Autodesk Inventor part; units mm, degrees
ref_plane "YZ Plane" through (0, 0, 0) normal (1, 0, 0) x (0, 1, 0)
ref_plane "XZ Plane" through (0, 0, 0) normal (0, 1, 0) x (-1, 0, 0)
ref_plane "XY Plane" through (0, 0, 0) normal (0, 0, 1) x (1, 0, 0)
sketch "Sketch1" plane through (0, 0, 0) normal (0, 0, 1) x (1, 0, 0)
  circle A0 centre (0, 0) radius 2.65
  circle A1 centre (0, 0) radius 3.5
  dimension "d0" = 5.3
  dimension "d1" = 7
extrude "Extrusion1" add sketch "Sketch1" along normal blind 15
sketch "Sketch2" plane through (0, 0, 15) normal (0, 0, 1) x (1, 0, 0)
  circle A0 centre (0, 0) radius 2.65
  circle A1 centre (0, 0) radius 3.75
  line L0 (-6, 0.85) -> (6, 0.85)
  line L1 (6, 0.85) -> (6, -0.85)
  line L2 (6, -0.85) -> (-6, -0.85)
  line L3 (-6, -0.85) -> (-6, 0.85)
  line L4 (-6, 0.85) -> (6, -0.85) construction
  line L5 (6, 0.85) -> (-6, -0.85) construction
  point P0 (-3.6524, 0.85)
  point P1 (-3.6524, -0.85)
  point P2 (3.6524, -0.85)
  point P3 (3.6524, 0.85)
  dimension "d4" = 7.5
  dimension "d5" = 12
  dimension "d6" = 1.7
extrude "Extrusion2" add sketch "Sketch2" along normal blind 25 contours A0 L0 A1 L2 | A0 L0 A1 | L2 A1 A0 | A0 L2 A1 L0 | L0 L1 L2 A1 | A1 L2 L3 L0
properties part number "final pin_3DPrint"
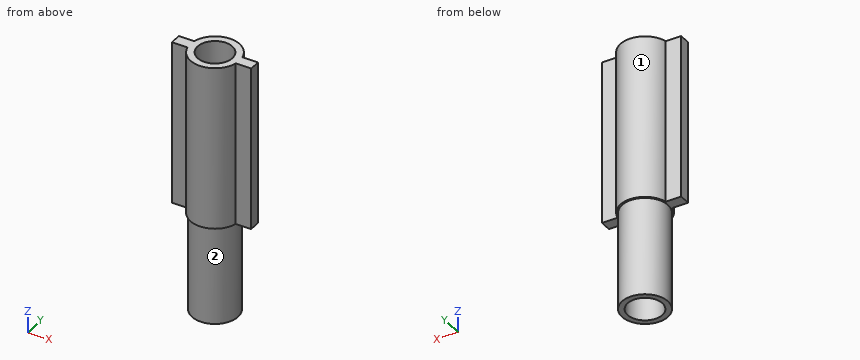
Could you check a few things on this model? Use its own coordinates, in mm. Face numbers are marked on the shaded views. A direction names the side the tool comes from. Round coordinates to 2 decimals unless told otherwise and drop trailing zeros. Order: outer loops, then holes, each group sorted by start corner. A loop starts at its lowest first (then second) coordinate and runs counter-clockwise, first axis right, second up.
(1) Imagine slicing it at A-A (y = 0). Write out the boundary of the cut face in (x, z).
Response values:
outline: (-6, 15) - (-3.5, 15) - (-3.5, 0) - (-2.65, 0) - (-2.65, 40) - (-6, 40) - close; (2.65, 0) - (3.5, 0) - (3.5, 15) - (6, 15) - (6, 40) - (2.65, 40) - close
(2) I'm going to push flat-ended pins straight in: pin 1 (3 mm diameter, centred on x = -1.5, z = 25.5, fed in from +Y); pin 2 (2 mm diameter, centred on x = 0.5, y = 1, fed in from -Z); pin 3 (0.7 mm diameter, centred on x = -4.5, z = 21.5, fed in from -Y); pin 4 (1.2 mm diameter, centred on x = -4.5, z = 25.5, fed in from +Y). Where does each tip first touch, or does it pass through?
Response values:
pin 1: stops at y = 3.75
pin 2: passes through
pin 3: stops at y = -0.85
pin 4: stops at y = 0.85
(3) Imagine slicing it at C-C (z = 21). Write out the boundary of the cut face in (x, y).
Response values:
outline: (-6, -0.85) - (-3.65, -0.85) arc R3.75 ccw to (3.65, -0.85) - (6, -0.85) - (6, 0.85) - (3.65, 0.85) arc R3.75 ccw to (-3.65, 0.85) - (-6, 0.85) - close; hole circle Ø5.3 at (0, 0)
(4) Imagine slicing it at B-B (x = 0). Write out the boundary of the cut face in (y, z).
Response values:
outline: (-3.75, 15) - (-3.5, 15) - (-3.5, 0) - (-2.65, 0) - (-2.65, 40) - (-3.75, 40) - close; (2.65, 0) - (3.5, 0) - (3.5, 15) - (3.75, 15) - (3.75, 40) - (2.65, 40) - close
(5) Imagine slicing it at D-D (z = 13). Write out the boundary of the cut face in (x, y).
Response values:
outline: circle Ø7 at (0, 0); hole circle Ø5.3 at (0, 0)
(6) Please list where these lines run through material, in increasing order: line 1 along Y through (x, z) = (0, 26); line 2 along Y through (x, z) = (0, 13); line 3 along Z through (x, y) = (-5, -0.5).
Response values:
line 1: y = -3.75 to -2.65, 2.65 to 3.75
line 2: y = -3.5 to -2.65, 2.65 to 3.5
line 3: z = 15 to 40
(7) Which directions (+Z, -Z, +X, -X, +Y, -Y) give clear straight access to the entire face, cutting with the end or side of a thin tool? Please do the marked faces 1 and 2.
Response values:
face 1: +Z, -Z, +Y
face 2: -Z
